Source: CAD feature listing. Evaluate the final solid. Frame: model axes, mm. Face numbers are marked on the shaded views. A direction names the side the tool comes from. Round coordinates to 2 decimals unless told otherwise and drop trailing zeros. Order: outer loops, then holes, each group sorted by start corner. A loop starts at its lowest first (then second) coordinate and runs counter-clockwise, first axis right, second up. Notation, with made-up numbers: M 37.25,35.25 L 79.25,35.25 A27 ccw 79.25,65.25 Z; hole C 29,2.25 d2. An arc over 180 degrees is marked long. Use one line per item in the form item = value. Start each with the question number.
Q1. Section B-B (x = 14). Return the cut outline in (y, z).
Q2. Material intervals for probe 1 along X at (y, z) = (-12, -9); probe 2 along Z at (x, y) = (-26, -28); probe 3 along X at (y, z) = (-27, -25), sorted ascending.
Q3. Pull-direction query (X, two-part tool) for the marked faces 1, 2, 3 and 4; classes: pulls with the +X half, pulls with the -X half, needs draft (parallel to the pull), parting line crosses it, or undercut.
Q4. Section A-A (z = -17). Return the cut outline in (x, y), plus the area to 3 significant figures.
Q5. Section D-D (y = -13.5). Return the cut outline in (x, z).
Q6. Contact query for flat-ended pins moving along their axis: pin 1 (1 mm diameter, centred on x = 10.5, z = -24, fed in from +Y); pin 2 (2 mm diameter, centred on y = -29, z = -6.5, fed in from +X); pin 3 (10 mm diameter, centred on y = -32.5, z = -29, fed in from +X). Output: stop coordinate, or through.
Q7. Section C-C (y = -19.5). Return the cut outline in (x, z), plus the area to 3 significant figures.
Q8. Reachability of the marked faces 5 and 6 from +Z, -Z, +X, -X, +Y, -Y: full face, straight path, thin tool, end or side. Return the list, or none.
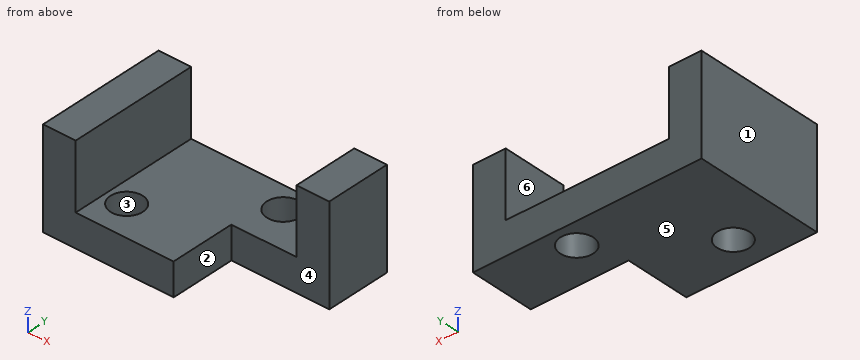
from build123d import *

# Parameters (mm, degrees)
F0_W      = 88.9
F0_H      = 38.1
F1_DEPTH  = 50.8
F2_W      = 63.5
F2_H      = 25.4
F3_DEPTH  = 50.8
F4_W      = 38.1
F4_H      = 25.4
F5_DEPTH  = 38.1
F6_W      = 12.7
F6_H      = 25.4
F7_DEPTH  = 38.1
F8_R      = 6.373614
F9_DEPTH  = 25.4
F10_R     = 6.283749
F11_DEPTH = 25.4


with BuildPart() as f1:
    # F0 (on Front) → F1 (new body)
    with BuildSketch(Plane.XZ):
        with Locations((1.654342, -16.239445)):
            Rectangle(F0_W, F0_H)
    extrude(amount=F1_DEPTH)

    # F2 (on face) → F3 (cut)
    with BuildSketch(Plane.XZ.offset(50.8)):
        with Locations((1.654342, -9.889445)):
            Rectangle(F2_W, F2_H)
    extrude(amount=-F3_DEPTH, mode=Mode.SUBTRACT)

    # F4 (on face) → F5 (cut)
    with BuildSketch(Plane.XY.offset(-22.589445)):
        with Locations((27.054342, -38.1)):
            Rectangle(F4_W, F4_H)
    extrude(amount=-F5_DEPTH, mode=Mode.SUBTRACT)

    # F6 (on face) → F7 (cut)
    with BuildSketch(Plane.XY.offset(2.810555)):
        with Locations((39.754342, -38.1)):
            Rectangle(F6_W, F6_H)
    extrude(amount=-F7_DEPTH, mode=Mode.SUBTRACT)

    # F8 (on face) → F9 (cut)
    with BuildSketch(Plane.XY.offset(-22.589445)):
        with Locations((14.187237, -9.558421)):
            Circle(F8_R)
    extrude(amount=-F9_DEPTH, mode=Mode.SUBTRACT)

    # F10 (on face) → F11 (cut)
    with BuildSketch(Plane.XY.offset(-22.589445)):
        with Locations((-21.933412, -37.581116)):
            Circle(F10_R)
    extrude(amount=-F11_DEPTH, mode=Mode.SUBTRACT)


solid = f1.part
Results list:
q1.outline = M -25.4,-35.29 L -15.93,-35.29 L -15.93,-22.59 L -25.4,-22.59 Z; M -3.19,-35.29 L 0,-35.29 L 0,-22.59 L -3.19,-22.59 Z
q2.probe_1 = -42.8 to -30.1, 33.4 to 46.1
q2.probe_2 = -35.29 to -22.59
q2.probe_3 = -42.8 to 8
q3.face_1 = pulls with the -X half
q3.face_2 = pulls with the +X half
q3.face_3 = undercut
q3.face_4 = needs draft
q4.outline = M -42.8,-50.8 L -30.1,-50.8 L -30.1,0 L -42.8,0 Z; M 33.4,-25.4 L 46.1,-25.4 L 46.1,0 L 33.4,0 Z
q4.area = 968 mm2
q5.outline = M -42.8,-35.29 L 9.18,-35.29 L 9.18,-22.59 L -30.1,-22.59 L -30.1,2.81 L -42.8,2.81 Z; M 19.2,-35.29 L 46.1,-35.29 L 46.1,2.81 L 33.4,2.81 L 33.4,-22.59 L 19.2,-22.59 Z
q6.pin_1 = 0
q6.pin_2 = -30.1
q6.pin_3 = 8
q7.outline = M -42.8,-35.29 L 46.1,-35.29 L 46.1,2.81 L 33.4,2.81 L 33.4,-22.59 L -30.1,-22.59 L -30.1,2.81 L -42.8,2.81 Z
q7.area = 1,770 mm2
q8.face_5 = -Z, +X, -X, +Y, -Y
q8.face_6 = +Z, +Y, -Y
